```python
from build123d import *

# Parameters (mm, degrees)
SKETCH1_W               = 24
SKETCH1_H               = 14.07
BOSS_EXTRUDE1_DEPTH     = 29.97
SKETCH2_W               = 22
SKETCH2_H               = 12.07
CUT_EXTRUDE1_DEPTH      = 28.97
CUT_EXTRUDE2_DEPTH      = 41.892123936
CUT_EXTRUDE2_DEPTH_BACK = 41.892123936
SKETCH3_W               = 12.07
SKETCH3_H               = 2.35


with BuildPart() as part:
    # Sketch1 → Boss-Extrude1 (new body)
    with BuildSketch(Plane(origin=(0, 0, 0), x_dir=(1, 0, 0), z_dir=(0, 1, 0))):
        with Locations((12, 7.035)):
            Rectangle(SKETCH1_W, SKETCH1_H)
    extrude(amount=BOSS_EXTRUDE1_DEPTH)

    # Sketch2 → Cut-Extrude1 (cut)
    with BuildSketch(Plane(origin=(0, 29.97, 0), x_dir=(1, 0, 0), z_dir=(0, 1, 0))):
        with Locations((12, 7.035)):
            Rectangle(SKETCH2_W, SKETCH2_H)
    extrude(amount=-CUT_EXTRUDE1_DEPTH, mode=Mode.SUBTRACT)

    # Sketch3 → Cut-Extrude2 (cut, two sides: drawn at the far end of the back side and taken through both)
    with BuildSketch(Plane.ZY.offset(-CUT_EXTRUDE2_DEPTH_BACK)):
        with Locations((-7.035, 17.645)):
            Rectangle(SKETCH3_W, SKETCH3_H)
    extrude(amount=CUT_EXTRUDE2_DEPTH + CUT_EXTRUDE2_DEPTH_BACK, mode=Mode.SUBTRACT)


solid = part.part
```
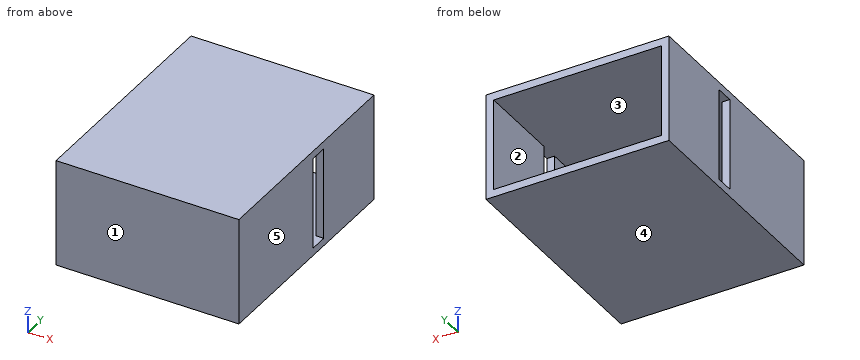
Geometry check sheet. Reference: the model listing, model coordinates, mm. Face numbers are marked on the shaded views. A direction names the side the tool comes from. Coordinates: 2 decimals unless noted, no trailing zeros. Loops run counter-clockwise (first coordinate to the right, second up) from the corner with the lowest first, then second, coordinate; pieces in that order, holes last. Notation, with made-up numbers: (12, -7) -> (40, -7) arc R31 cw to (40, 27) -> close; hole circle Ø10 at (31.25, -38). An arc over 180 degrees is marked (long way). Put each result on its own line as item: value.
1) Gauge pin test, flat end, axial feed: pin 1 Ø6 at (x, z) = (10, -10) entering from +Y. Record the tip position at first contact, or that the pin passes through.
Result set:
pin 1: stops at y = 1
2) Thickness scan on line 1 (Z direction, x = 20.75, y = 17.5); line 2 (X direction, y = 28, z = -7.75); line 3 (Y direction, x = 10.25, z = -5.25). Record the ranges inside material, lowest first.
Result set:
line 1: z = -14.07 to -13.07, -1 to 0
line 2: x = 0 to 1, 23 to 24
line 3: y = 0 to 1
3) Cross-section at C-C on x = 11.25. Record the boundary of the cut face in (y, z), plus the area to 3 significant figures.
Result set:
outline: (0, -14.07) -> (29.97, -14.07) -> (29.97, -13.07) -> (1, -13.07) -> (1, -1) -> (29.97, -1) -> (29.97, 0) -> (0, 0) -> close
area: 72.0 mm^2
4) Tool access check on the marked faces 1 and 2. Record the directions out of +Z, -Z, +X, -X, +Y, -Y that give a thin tool (end or side, any length) a straight path to the whole face; none if there is none.
Result set:
face 1: +Z, -Z, +X, -X, -Y
face 2: +Y
5) Cross-section at B-B on y = 9.5. Record the boundary of the cut face in (x, z).
Result set:
outline: (0, -14.07) -> (24, -14.07) -> (24, 0) -> (0, 0) -> close; hole (1, -13.07) -> (23, -13.07) -> (23, -1) -> (1, -1) -> close
6) Cross-section at A-A on z = -5.5. Record the boundary of the cut face in (x, y).
Result set:
outline: (0, 0) -> (24, 0) -> (24, 16.47) -> (23, 16.47) -> (23, 1) -> (1, 1) -> (1, 16.47) -> (0, 16.47) -> close; (0, 18.82) -> (1, 18.82) -> (1, 29.97) -> (0, 29.97) -> close; (23, 18.82) -> (24, 18.82) -> (24, 29.97) -> (23, 29.97) -> close
7) Release check for a two-part mould opening along X. For the marked faces 3, 4 and 5 record: released by +X, released by -X, zero draft, split by the parting line, or undercut.
Result set:
face 3: undercut
face 4: zero draft
face 5: released by +X
